Source: CAD feature listing. Evaluate the final solid. Frame: model axes, mm. A direction names the side the tool comes from. Round coordinates to 2 decimals unless told otherwise and drop trailing zeros. Order: outer loops, then holes, each group sorted by start corner. A loop starts at its lowest first (then second) coordinate and runs counter-clockwise, first axis right, second up. Notation, with made-up numbers: M 17,-21 L 43,-21 A21 ccw 43,-17 Z; hole C 70.25,10.25 d3. An arc over 180 degrees is marked long. Answer in a Markdown table with one row per item. Add a question column.
```python
from build123d import *

# Parameters (mm, degrees)
F0_W      = 127
F0_H      = 127
F1_DEPTH  = 127
F2_R      = 12.7
F3_DEPTH  = 6.35
F4_R      = 12.7
F5_DEPTH  = 6.35
F6_R      = 11.1125
F7_DEPTH  = 6.35
F8_R      = 12.7
F9_DEPTH  = 6.35
F10_R     = 12.7
F10_R_2   = 12.703885
F11_DEPTH = 6.35
F12_R     = 12.7
F13_DEPTH = 6.35


with BuildPart() as f1:
    # F0 (on Top) → F1 (new body)
    with BuildSketch(Plane.XY):
        Rectangle(F0_W, F0_H)
    extrude(amount=F1_DEPTH)

    # F2 (on face) → F3 (cut)
    with BuildSketch(Plane.XY.offset(127)):
        Circle(F2_R)
    extrude(amount=-F3_DEPTH, mode=Mode.SUBTRACT)

    # F4 (on face) → F5 (cut)
    with BuildSketch(Plane.XZ.offset(63.5)):
        with Locations((-41.275, 22.225)):
            Circle(F4_R)
        with Locations((41.275, 104.775)):
            Circle(F4_R)
    extrude(amount=-F5_DEPTH, mode=Mode.SUBTRACT)

    # F6 (on face) → F7 (cut)
    with BuildSketch(Plane.YZ.offset(63.5)):
        with Locations((-41.275, 22.225)):
            Circle(F6_R)
        with Locations((41.275, 104.775)):
            Circle(F6_R)
        with Locations((0, 63.5)):
            Circle(F6_R)
    extrude(amount=-F7_DEPTH, mode=Mode.SUBTRACT)

    # F8 (on face) → F9 (cut)
    with BuildSketch(Plane(origin=(-63.5, 0, 0), x_dir=(0, -1, 0), z_dir=(-1, 0, 0))):
        with Locations((-41.275, 22.225)):
            Circle(F8_R)
        with Locations((41.275, 22.225)):
            Circle(F8_R)
        with Locations((41.275, 104.775)):
            Circle(F8_R)
        with Locations((-41.275, 104.775)):
            Circle(F8_R)
    extrude(amount=-F9_DEPTH, mode=Mode.SUBTRACT)

    # F10 (on face) → F11 (cut)
    with BuildSketch(Plane(origin=(0, 63.5, 0), x_dir=(-1, 0, 0), z_dir=(0, 1, 0))):
        with Locations((-41.275, 104.775)):
            Circle(F10_R)
        with Locations((41.275, 104.775)):
            Circle(F10_R)
        with Locations((41.275, 22.225)):
            Circle(F10_R_2)
        with Locations((-37.138888, 26.361112)):
            Circle(F10_R)
        with Locations((0, 63.5)):
            Circle(F10_R)
    extrude(amount=-F11_DEPTH, mode=Mode.SUBTRACT)

    # F12 (on face) → F13 (cut)
    with BuildSketch(Plane(origin=(0, 0, 0), x_dir=(1, 0, 0), z_dir=(0, 0, -1))):
        with Locations((-41.275, 41.275)):
            Circle(F12_R)
        with Locations((41.275, 41.275)):
            Circle(F12_R)
        with Locations((-41.275, 0)):
            Circle(F12_R)
        with Locations((-41.275, -41.275)):
            Circle(F12_R)
        with Locations((41.275, 0)):
            Circle(F12_R)
        with Locations((41.275, -41.275)):
            Circle(F12_R)
    extrude(amount=-F13_DEPTH, mode=Mode.SUBTRACT)


solid = f1.part
```
(1) Draft query along Y for faces 6 (the face through (-31.194, 60.369, 14.495)), 7 (the face through (-2.75, -12.4, 123.87)), 8 (the face through (41, -57.15, 105)). Return one class per face: +Y half, -Y half, draft (parallel to the pull), parting line (faces both ways), or undercut.
(2) Access query for faces 1 (the face through (60.369, -1.447, 74.518)), 2 (the face through (39.622, -60.369, 117.367)), 3 (the face through (-57.15, 41, 22)), 4 (the face through (-29.543, -36.411, 3.131)), 5 (the face through (-39.622, 60.369, 117.367)). Directions: +Z, -Z, +X, -X, +Y, -Y. A direction counts if a zero-diameter tool reaches every point of the face in a straight line with its end or side. Return the directions, or none.
(3) Cut plane C-C (x = 0). Return loops of the section in (y, z).
(4) Cut plane D-D (y = -36). Return loops of the section in (x, z).
(5) Line query: line 1 (Y direction, x = -58, z = 28); line 2 (Y direction, x = -36.5, z = 106); line 3 (Z direction, x = 4, y = -2). Output: solid intervals per line, ascending. Write a range as from..to.
(6) Pin query (flat end, axial travel): pin 1 (2 mm diameter, centred on x = -32, z = 22.5, fed in from +Y); pin 2 (7.5 mm diameter, centred on x = -39.5, z = 21.5, fed in from -Y); pin 3 (7.5 mm diameter, centred on x = 47, y = -35, fed in from -Z). Return the tip coordinate at first contact, or that it passes through.
(7) Cut plane A-A (z = 63.5). Return loops of the section in (x, y), and give its area (3 significant figures).
Answer list:
| question | item | result |
|---|---|---|
| 1 | face 6 | draft |
| 1 | face 7 | undercut |
| 1 | face 8 | -Y half |
| 2 | face 1 | +X |
| 2 | face 2 | -Y |
| 2 | face 3 | -X |
| 2 | face 4 | -Z |
| 2 | face 5 | +Y |
| 3 | outline | M -63.5,0 L 63.5,0 L 63.5,50.8 L 57.15,50.8 L 57.15,76.2 L 63.5,76.2 L 63.5,127 L 12.7,127 L 12.7,120.65 L -12.7,120.65 L -12.7,127 L -63.5,127 Z |
| 4 | outline | M -63.5,0 L -52.83,0 L -52.83,6.35 L -29.72,6.35 L -29.72,0 L 29.72,0 L 29.72,6.35 L 52.83,6.35 L 52.83,0 L 63.5,0 L 63.5,12.44 L 57.15,12.44 L 57.15,32.01 L 63.5,32.01 L 63.5,127 L -63.5,127 L -63.5,116.33 L -57.15,116.33 L -57.15,93.22 L -63.5,93.22 L -63.5,33.78 L -57.15,33.78 L -57.15,10.67 L -63.5,10.67 Z |
| 5 | line 1 | -63.5..-52.59, -29.96..29.96, 52.59..63.5 |
| 5 | line 2 | -63.5..57.15 |
| 5 | line 3 | 0..120.65 |
| 6 | pin 1 | y = 57.15 |
| 6 | pin 2 | y = -57.15 |
| 6 | pin 3 | z = 6.35 |
| 7 | outline | M -63.5,-63.5 L 63.5,-63.5 L 63.5,-11.11 L 57.15,-11.11 L 57.15,11.11 L 63.5,11.11 L 63.5,63.5 L 12.7,63.5 L 12.7,57.15 L -12.7,57.15 L -12.7,63.5 L -63.5,63.5 Z |
| 7 | area | 15,800 mm² |
